```python
from build123d import *

# Parameters (mm, degrees)
EXTRUDE_1_DEPTH           = 10
HOLE_WIZARD_8_0_8_1_D     = 8
HOLE_WIZARD_8_0_8_1_DEPTH = 6.25
HOLE_WIZARD_M41_D         = 4.5
HOLE_WIZARD_M41_DEPTH     = 11
HOLE_WIZARD_M41_TIP       = 1.351936393
HOLE_WIZARD_M42_D         = 4.5
HOLE_WIZARD_M42_DEPTH     = 6.25
M4X0_72_D                 = 3.3
FILLET_2_R                = 10
FILLET_3_R                = 2


with BuildPart() as part:
    # Эскиз1 → Бобышка-Вытянуть1 (new body)
    with BuildSketch(Plane(origin=(0, 0, 0), x_dir=(1, 0, 0), z_dir=(0, 1, 0))):
        with BuildLine():
            Line((67.173762079, -7), (7.826237921, -7))
            ThreePointArc((7.826237921, -7), (-9.585144756, -4.28660705), (0, 10.5))
            Line((0, 10.5), (75, 10.5))
            ThreePointArc((75, 10.5), (84.585144756, -4.28660705), (67.173762079, -7))
        make_face()
        with BuildLine():
            Line((7.462405778, -0.75), (67.537594222, -0.75))
            ThreePointArc((67.537594222, -0.75), (82.5, 0), (67.537594222, 0.75))
            Line((67.537594222, 0.75), (7.462405778, 0.75))
            ThreePointArc((7.462405778, 0.75), (-7.5, 0), (7.462405778, -0.75))
        make_face(mode=Mode.SUBTRACT)
    extrude(amount=EXTRUDE_1_DEPTH)

    # Диаметр отверстия Ø8.0 (8)1
    with Locations(Plane.XY.offset(7)):
        with Locations((27.5, 5), (47.5, 5)):
            Hole(HOLE_WIZARD_8_0_8_1_D / 2, depth=HOLE_WIZARD_8_0_8_1_DEPTH)

    # Отверстие с зазором M41
    with Locations(Plane.XY.offset(-0.75)):
        with Locations((47.5, 5), (27.5, 5)):
            Hole(HOLE_WIZARD_M41_D / 2, depth=HOLE_WIZARD_M41_DEPTH)
            with Locations((0, 0, -(HOLE_WIZARD_M41_DEPTH + HOLE_WIZARD_M41_TIP / 2))):  # 118° drill point
                Cone(0, HOLE_WIZARD_M41_D / 2, HOLE_WIZARD_M41_TIP, mode=Mode.SUBTRACT)

    # Отверстие с зазором M42
    with Locations(Plane.XY.offset(7)):
        with Locations((37.5, 5)):
            Hole(HOLE_WIZARD_M42_D / 2, depth=HOLE_WIZARD_M42_DEPTH)

    # Отверстие обработанное метчиком M4x0.72 (through all)
    with Locations(Plane.XY.offset(-0.75)):
        with Locations((37.5, 5)):
            Hole(M4X0_72_D / 2)

    # Скругление2
    fillet_2_edges = [part.edges().sort_by_distance(p)[0] for p in [
        (67.173762079, 5, 7),
        (7.826237921, 5, 7),
    ]]
    fillet(fillet_2_edges, radius=FILLET_2_R)

    # Скругление3
    fillet_3_edges = [part.edges().sort_by_distance(p)[0] for p in [
        (7.462405778, 5, -0.75),
        (7.462405778, 5, 0.75),
        (67.537594222, 5, 0.75),
        (67.537594222, 5, -0.75),
    ]]
    fillet(fillet_3_edges, radius=FILLET_3_R)


solid = part.part
```
Here's how the part is built. I have some questions about the finished solid (model axes, mm). A direction names the side the tool comes from. Give positions to 0.01 mm unless a question says otherwise; leave off trailing zeros. Write each loop counter-clockwise with the first axis right and the second up, starting at its lowest first coordinate (ties: lowest second). Pieces come first, ordered by that corner, then holes. Notation, with made-up numbers: (47.5, -2.75) -> (87.5, -2.75) arc R33 ccw to (87.5, 30.25) -> close; hole circle Ø2 at (-13.75, -36). An arc over 180 degrees is marked (long way). Write each question's results on one line, items separated by ' | '.
Item 1: Suppose I cut it at D-D on x = 47.5. Write out the boundary of the cut face in (y, z), plus the area to 3 significant figures.
Output:
outline: (0, -10.5) -> (2.75, -10.5) -> (2.75, -0.75) -> (0, -0.75) -> close; (0, 0.75) -> (1, 0.75) -> (1, 7) -> (0, 7) -> close; (7.25, -10.5) -> (10, -10.5) -> (10, -0.75) -> (7.25, -0.75) -> close; (9, 0.75) -> (10, 0.75) -> (10, 7) -> (9, 7) -> close | area: 66.1 mm^2
Item 2: For pin 1 Ø1.5 at (y, z) = (1.5, -2) entering from -X; pin 2 Ø4 at (x, y) = (37.5, 5) entering from +Z; pin 3 Ø2 at (x, z) = (5.5, -2) entering from -Y; pin 4 Ø5 at (x, y) = (47.5, 5) entering from -Z, each with a flat end and sliding along its axis, tell me the tip position at first contact or that it passes through.
Output:
pin 1: stops at x = -10.43 | pin 2: stops at z = -0.75 | pin 3: passes through | pin 4: stops at z = -10.5
Item 3: On a 3-axis mill with a long thin cutter (end or side, diameter ignored), from which of +Z, -Z, +X, -X, +Y, -Y can I reach the whole of each face in a straight line? I mean faces 4 (the face through (67.11, 5.07, 1.15)), 5 (the face through (50.7, 2.6, 3.8)), 6 (the face through (38, 2, 7)), 7 (the face through (38, 10, -2)), 8 (the face through (38, 0, -2)). Say none if no direction works.
Output:
face 4: +Y, -Y | face 5: +Z | face 6: +Z, +Y, -Y | face 7: +Z, -Z, +X, -X, +Y | face 8: +Z, -Z, +X, -X, -Y
Item 4: We'd pull the mould along Z, two halves only. Please class faces 1 (the face through (-7.494, 4.93, -0.299)), 2 (the face through (37, 3, -10.5)), 3 (the face through (39.15, 5.07, -5.69)): pulls with the +Z half, pulls with the -Z half, needs draft (parallel to the pull), parting line crosses it, or undercut.
Output:
face 1: undercut | face 2: pulls with the -Z half | face 3: needs draft
Item 5: Suppose I cut it at A-A on x = 20. Write out the boundary of the cut face in (y, z), plus the area to 3 significant figures.
Output:
outline: (0, -10.5) -> (10, -10.5) -> (10, -0.75) -> (0, -0.75) -> close; (0, 0.75) -> (10, 0.75) -> (10, 7) -> (0, 7) -> close | area: 160 mm^2
Item 6: Suppose I cut it at B-B on x = 37.5. Write out the boundary of the cut face in (y, z), plus the area to 3 significant figures.
Output:
outline: (0, -10.5) -> (3.35, -10.5) -> (3.35, -0.75) -> (0, -0.75) -> close; (0, 0.75) -> (2.75, 0.75) -> (2.75, 7) -> (0, 7) -> close; (6.65, -10.5) -> (10, -10.5) -> (10, -0.75) -> (6.65, -0.75) -> close; (7.25, 0.75) -> (10, 0.75) -> (10, 7) -> (7.25, 7) -> close | area: 99.7 mm^2
Item 7: If I drill on L1, parallel to Z at x = 14, y = 4; L2, parallel to Y at x = 27.5, z = -4.25; L3, parallel to X at y = 9.5, z = 1.25, over which ranges is the centre line in solid material (lowest first)?
Output:
L1: z = -10.5 to -0.75, 0.75 to 7 | L2: y = 0 to 2.75, 7.25 to 10 | L3: x = -10.43 to -7.4, 7.77 to 67.23, 82.4 to 85.43
Item 8: Suppose I cut it at C-C on z = 3.75. Write out the boundary of the cut face in (x, y).
Output:
outline: (-9.81, 0) -> (-6.5, 0) -> (-6.5, 10) -> (-9.81, 10) -> close; (6.5, 0) -> (68.5, 0) -> (68.5, 10) -> (6.5, 10) -> close; (81.5, 0) -> (84.81, 0) -> (84.81, 10) -> (81.5, 10) -> close; hole circle Ø8 at (27.5, 5); hole circle Ø4.5 at (37.5, 5); hole circle Ø8 at (47.5, 5)
